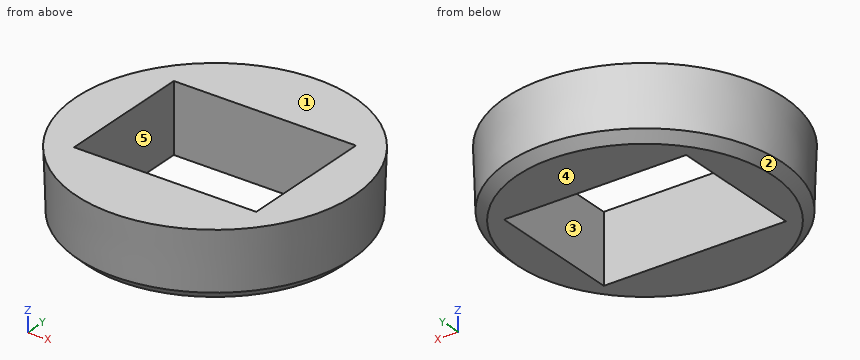
```python
from build123d import *

# Parameters (mm, degrees)
CHAMFER_SIZE = 2
SKETCH001_W  = 40
SKETCH001_H  = 30
POCKET_DEPTH = 15.001


with BuildPart() as part:
    # Sketch → Revolution (revolve)
    with BuildSketch(Plane.XZ):
        Polygon((0, 0), (30, 0), (30.5, 15), (0, 15), align=None)
    revolve(axis=Axis((0, 0, 0), (0, 0, 1)))

    # Chamfer
    chamfer_edges = [part.edges().sort_by_distance(p)[0] for p in [
        (-30, 0, 0),
    ]]
    chamfer(chamfer_edges, length=CHAMFER_SIZE)

    # Sketch001 (on Face4 of Chamfer) → Pocket (cut, through all)
    with BuildSketch(Plane(origin=(0, 0, 15), x_dir=(-1, 0, 0), z_dir=(0, 0, 1))):
        Rectangle(SKETCH001_W, SKETCH001_H)
    extrude(amount=-POCKET_DEPTH, mode=Mode.SUBTRACT)


solid = part.part
```
Geometry check sheet. Reference: the model listing, model coordinates, mm. Face numbers are marked on the shaded views. A direction names the side the tool comes from. Give positions to 0.01 mm unless a question says otherwise; leave off trailing zeros. Loops run counter-clockwise (first coordinate to the right, second up) from the corner with the lowest first, then second, coordinate; pieces in that order, holes last. Notation, with made-up numbers: M 32.5,-11.75 L 81.5,-11.75 A33 ccw 81.5,19.25 Z; hole C 86,5 d2. An arc over 180 degrees is marked long. Write item = value, one per line.
(1) Sectioned sample at B-B, the plane x = 0. Record the cut outline in (y, z).
Answer below:
outline = M -30.5,15 L -30.07,2 L -28,0 L -15,0 L -15,15 Z; M 15,0 L 28,0 L 30.07,2 L 30.5,15 L 15,15 Z
(2) Tool access check on the marked faces 4 and 5. Record the directions out of +Z, -Z, +X, -X, +Y, -Y that give a thin tool (end or side, any length) a straight path to the whole face; none if there is none.
Answer below:
face_4 = -Z, +X, -X, +Y, -Y
face_5 = +Z, -Z
(3) Sectioned sample at D-D, the plane z = 9.25. Record the cut outline in (x, y).
Answer below:
outline = C 0,0 d60.62; hole M -20,-15 L 20,-15 L 20,15 L -20,15 Z
(4) Material ranges on line 1 (X direction, y = -4, z = 6.5); line 2 (Y direction, x = -15.5, z = 3.25); line 3 (Y direction, x = -10.5, z = 4.25), recorded low to high. Write a range as [from, to].
Answer below:
line_1 = [-29.95, -20], [20, 29.95]
line_2 = [-25.81, -15], [15, 25.81]
line_3 = [-28.25, -15], [15, 28.25]
(5) Gauge pin test, flat ends, axial feed: pin 1 Ø6 at (x, z) = (7, 8.5) entering from +Y; pin 2 Ø4.5 at (y, z) = (4, 5) entering from +X; pin 3 Ø5 at (y, z) = (7, 13.5) entering from -X (3 decimals). Record the tip position at first contact, or that the pin passes through.
Answer below:
pin_1 = 30.03
pin_2 = 30.13
pin_3 = -30.125
(6) Sectioned sample at C-C, the plane z = 4.75. Record the cut outline in (x, y).
Answer below:
outline = C 0,0 d60.32; hole M -20,-15 L 20,-15 L 20,15 L -20,15 Z
(7) Sectioned sample at A-A, the plane y = 0. Record the cut outline in (x, z), plus the area to 3 significant figures.
Answer below:
outline = M -30.5,15 L -30.07,2 L -28,0 L -20,0 L -20,15 Z; M 20,0 L 28,0 L 30.07,2 L 30.5,15 L 20,15 Z
area = 304 mm2
(8) Release check for a two-part mould opening along Y. For the marked faces 1, 2 and 3 record: released by +Y, released by -Y, zero draft, split by the parting line, or undercut.
Answer below:
face_1 = zero draft
face_2 = split by the parting line
face_3 = undercut
